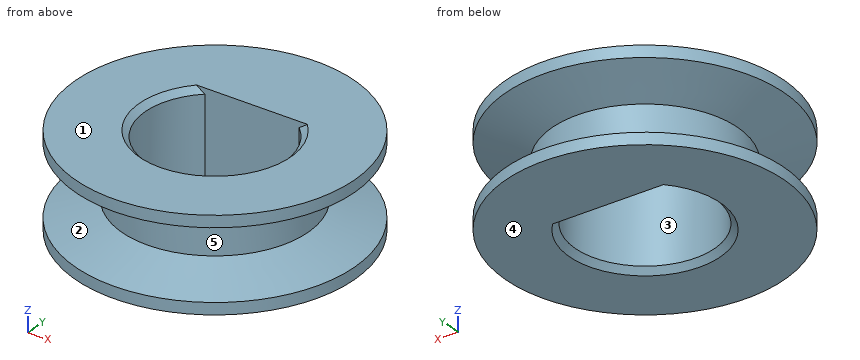
from build123d import *

# Parameters (mm, degrees)
SKETCH1_R           = 19.05
SKETCH1_R_2         = 9.525
EXTRUDE1_DEPTH      = 6.35
CHAMFER1_SIZE       = 0.79375
BOSS_EXTRUDE1_DEPTH = 12.7


with BuildPart() as part:
    # Sketch1 → Extrude1 (new, symmetric)
    with BuildSketch(Plane.XY):
        Circle(SKETCH1_R)
        Circle(SKETCH1_R_2, mode=Mode.SUBTRACT)
    extrude(amount=EXTRUDE1_DEPTH, both=True)

    # Chamfer1
    chamfer1_edges = [part.edges().sort_by_distance(p)[0] for p in [
        (-9.525, 0, -6.35),
        (-9.525, 0, 6.35),
    ]]
    chamfer(chamfer1_edges, length=CHAMFER1_SIZE)

    # Sketch2 → Cut-Revolve1 (revolve, cut)
    with BuildSketch(Plane(origin=(0, 0, 0), x_dir=(0, 0, -1), z_dir=(1, 0, 0)), mode=Mode.PRIVATE) as cut_revolve1_sk:
        Polygon((-4.7625, 19.05), (4.7625, 19.05), (2.451289012, 12.7), (-2.451289012, 12.7), align=None)
    revolve(cut_revolve1_sk.sketch.rotate(Axis((0, 0, 6.35), (0, 0, -1)), 180), axis=Axis((0, 0, 6.35), (0, 0, -1)), mode=Mode.SUBTRACT)

    # Sketch3 → Boss-Extrude1 (add, through all)
    with BuildSketch(Plane(origin=(0, 0, -6.35), x_dir=(-1, 0, 0), z_dir=(0, 0, -1))):
        with BuildLine():
            ThreePointArc((7.558172832, 7.025), (0, 10.31875), (-7.558172832, 7.025))
            Line((-7.558172832, 7.025), (7.558172832, 7.025))
        make_face()
    extrude(amount=-BOSS_EXTRUDE1_DEPTH)


solid = part.part
Part model, mm, in its own coordinate system. Face numbers are marked on the shaded views. A direction names the side the tool comes from. Coordinates: 2 decimals unless noted, no trailing zeros. Write each loop counter-clockwise with the first axis right and the second up, starting at its lowest first coordinate (ties: lowest second). Pieces come first, ordered by that corner, then holes. Notation, with made-up numbers: M 67,5.25 L 115,5.25 A21 cw 115,13.25 Z; hole C 28,-15.75 d10. An arc over 180 degrees is marked long. Return JSON: item names as keys, results as strings.
1. Flat gauge pins, fed straight in: pin 1 Ø2 at (y, z) = (-7.5, -1) entering from -X; pin 2 Ø6 at (x, y) = (9, 5) entering from +Z. Where does each tip first touch, or does it go through?
Determined:
{"pin 1": "x = -10.91", "pin 2": "z = 6.35"}
2. 3-axis set-ups, long thin cutter, end or side, ignore diameter. For the marked faces 4 and 5: which of +Z, -Z, +X, -X, +Y, -Y reach the whole face in a straight line?
Determined:
{"face 4": "-Z, +X, -X, +Y, -Y", "face 5": "none"}
3. Probe L1, parallel to X at y = 0, z = -1 (3 decimals); L2, parallel to X at y = 11, z = 1.75; L3, parallel to Z at x = 9, y = 16. List the from-to ranges inside material, lowest first.
Determined:
{"L1": "-12.7 to -9.525, 9.525 to 12.7", "L2": "-6.35 to 6.35", "L3": "-6.35 to -4.51, 4.51 to 6.35"}
4. Saw through at C-C, the plane z = -0.5. Write the cut outline in (x, y) (3 decimals), then the cut area to 3 significant figures.
Determined:
{"outline": "C 0,0 d25.4; hole M -6.432,7.025 A9.525 ccw long 6.432,7.025 Z", "area": "244 mm²"}
5. Pull direction X, two halves, no side cores. Call the marked faces 1, 2 and 3: pulls with the +X half, pulls with the -X half, needs draft (parallel to the pull), parting line crosses it, or undercut.
Determined:
{"face 1": "needs draft", "face 2": "parting line crosses it", "face 3": "undercut"}
